The model under review builds one solid part; all positions refer to its coordinate system, in mm. Face numbers are marked on the shaded views. Round coordinates to 2 decimals unless told otherwise and drop trailing zeros. Write each loop counter-clockwise with the first axis right and the second up, starting at its lowest first coordinate (ties: lowest second). Pieces come first, ordered by that corner, then holes. Notation, with made-up numbers: (86.5, 51.5) - (91.5, 51.5) arc R17 cw to (91.5, 64.5) - close; hole circle Ø7 at (86.25, 66). An arc over 180 degrees is marked (long way). Use one line per item in the form item = value.
from build123d import *

# Parameters (mm, degrees)
SKETCH_1_R          = 10.5
EXTRUDE_1_DEPTH     = 7
SKETCH_2_R          = 6
CUT_EXTRUDE_1_DEPTH = 17.416455159
SKETCH_3_R          = 9.3
SKETCH_3_R_2        = 7.2
CUT_EXTRUDE_2_DEPTH = 5.5
SWEEP_1_PROFILE_R   = 0.75


with BuildPart() as part:
    # 草图1 → 凸台-拉伸1 (new body)
    with BuildSketch(Plane.XY):
        Circle(SKETCH_1_R)
    extrude(amount=EXTRUDE_1_DEPTH)

    # 草图2 → 切除-拉伸1 (cut, through all)
    with BuildSketch(Plane.XY.offset(7)):
        Circle(SKETCH_2_R)
    extrude(amount=-CUT_EXTRUDE_1_DEPTH, mode=Mode.SUBTRACT)

    # 草图3 → 切除-拉伸2 (cut)
    with BuildSketch(Plane.XY.offset(7)):
        Circle(SKETCH_3_R)
        Circle(SKETCH_3_R_2, mode=Mode.SUBTRACT)
    extrude(amount=-CUT_EXTRUDE_2_DEPTH, mode=Mode.SUBTRACT)

    # 切除-扫描1: sweep along a path in 草图5
    with BuildLine(Plane.XY.offset(5.5)) as sweep_1_path:
        CenterArc((0, 0), 6, 0, 360)
    # 切除-扫描1 profile (on start of the path) → 切除-扫描1 (sweep, cut)
    with BuildSketch(Plane(origin=(6, 0, 5.5), x_dir=(0, 0, 1), z_dir=(0, 1, 0))):
        Circle(SWEEP_1_PROFILE_R)
    sweep(path=sweep_1_path.line, mode=Mode.SUBTRACT)


solid = part.part
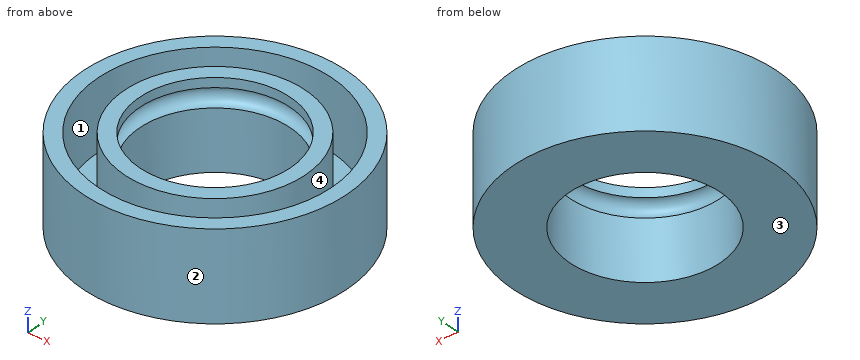
(1) To check wall thickness, follow L1, parallel to Y at x = 0, z = 6.85; L2, parallel to X at y = 3, z = 3.5; L3, parallel to X at y = -2.5, z = 5. State the ranges of each line that lie inside material, in increasing order.
Geometry results:
L1 = -10.5 to -9.3, -7.2 to -6, 6 to 7.2, 9.3 to 10.5
L2 = -10.06 to -8.8, -6.55 to -5.2, 5.2 to 6.55, 8.8 to 10.06
L3 = -10.2 to -8.96, -6.75 to -6.06, 6.06 to 6.75, 8.96 to 10.2
(2) Add section D-D on y = -8. Write out the cut boundary in (x, z).
Geometry results:
outline = (-6.8, 0) - (6.8, 0) - (6.8, 7) - (4.74, 7) - (4.74, 1.5) - (-4.74, 1.5) - (-4.74, 7) - (-6.8, 7) - close
(3) Add section B-B on z = 5.5. Write out the cut boundary in (x, y), then the cut area to 3 significant figures.
Geometry results:
outline = circle Ø21 at (0, 0); circle Ø14.4 at (0, 0); hole circle Ø18.6 at (0, 0); hole circle Ø13.5 at (0, 0)
area = 94.4 mm2
(4) The part is to be moulded in two halves that separate along Y. For the marked faces 1, 2, 3 and 4, say which applies: +Y half, -Y half, draft (parallel to the pull), parting line (faces both ways), or undercut.
Geometry results:
face_1 = undercut
face_2 = parting line
face_3 = draft
face_4 = undercut
(5) Add section A-A on x = 0. Write out the cut boundary in (y, z).
Geometry results:
outline = (-10.5, 0) - (-6, 0) - (-6, 4.75) arc R0.75 cw to (-6, 6.25) - (-6, 7) - (-7.2, 7) - (-7.2, 1.5) - (-9.3, 1.5) - (-9.3, 7) - (-10.5, 7) - close; (6, 0) - (10.5, 0) - (10.5, 7) - (9.3, 7) - (9.3, 1.5) - (7.2, 1.5) - (7.2, 7) - (6, 7) - (6, 6.25) arc R0.75 cw to (6, 4.75) - close
(6) Insertion check: P1, Ø3, axis at x = -3.5, z = 2.5, coming from the -Y side; P2, Ø1.5, axis at y = 7, z = 1, coming from the -X side; P3, Ø2, axis at x = -7.5, z = 6, coming from the -Y side. Each pin has a flat end and moves straight along its axis. Give the tip position at first contact, or say it passes through.
Geometry results:
P1 = -10.31
P2 = -8.44
P3 = -8.25
